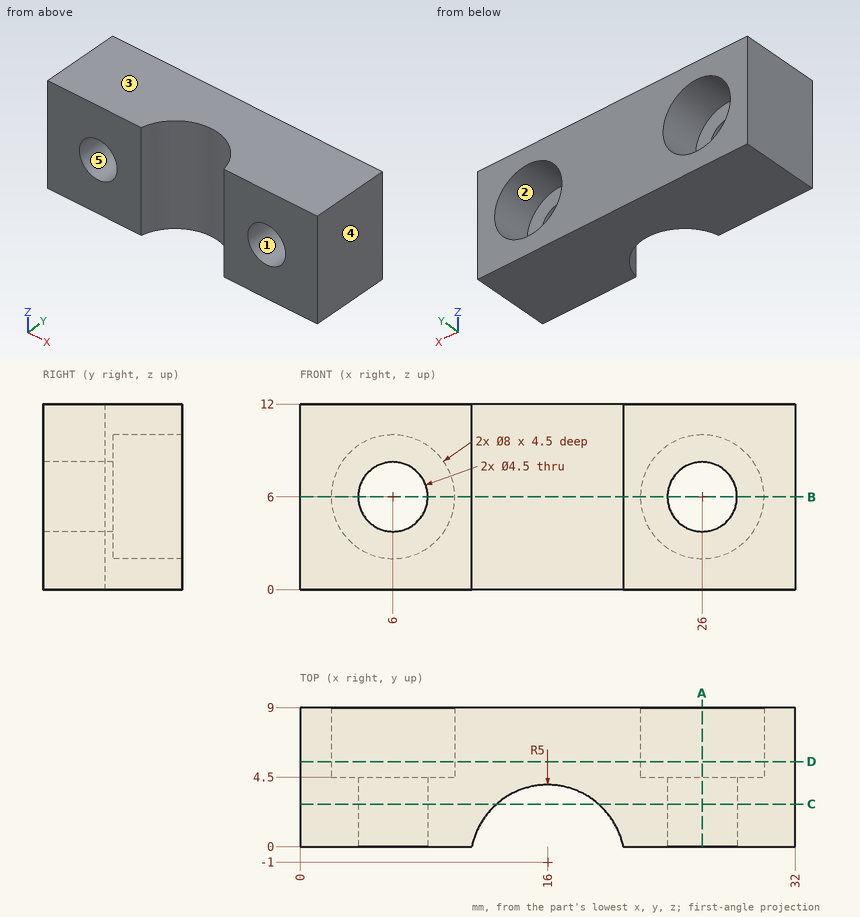
Geometry check sheet. Reference: drawing and pictorial views, mm from the part's lowest x, y, z. A direction names the side the tool comes from. Coordinates: 2 decimals unless noted, no trailing zeros. Write each loop counter-clockwise with the first axis right and the second up, starting at its lowest first coordinate (ties: lowest second). Pieces come first, ordered by that corner, then holes. Notation, with made-up numbers: (45.25, -27.5) - (74.25, -27.5) arc R19 cw to (74.25, -23.5) - close; hole circle Ø11 at (34.5, 32). An arc over 180 degrees is marked (long way). One line per question, with ' | ' between items. Start each with the question number.
1. Gauge pin test, flat end, axial feed: P1, Ø2.5, axis at x = 28, z = 5, coming from the +Y side. Record the tip position at first contact, or that the pin passes through.
2. Draft check along Z on the marked faces 3, 4 and 5. Enter one of: released by +Z, released by -Z, zero draft, split by the parting line, or undercut.
3. Access from +Z, -Z, +X, -X, +Y, -Y to the whole of each face (thin tool, end or side, straight path). Record for the marked faces 1 and 2.
4. Section check A-A (x = 26). Enter the section's corners in (y, z), plus the area to 4 significant figures.
5. Section check C-C (y = 2.75). Enter the section's corners in (x, z), plus the area to 3 significant figures.
6. Section check D-D (y = 5.5). Enter the section's corners in (x, z), plus the area to 3 significant figures.
7. Section check B-B (z = 6). Enter the section's corners in (x, y).
8. Material ranges on line 1 along X through (y, z) = (5.9, 6); line 2 along Z through (x, y) = (6, 2.75); line 3 along Z through (x, y) = (6, 6.75), recorded low to high.
Computed values:
1) P1: y = 4.5
2) face 3: released by +Z | face 4: zero draft | face 5: undercut
3) face 1: +Y, -Y | face 2: +Y
4) outline: (0, 0) - (9, 0) - (9, 2) - (4.5, 2) - (4.5, 3.75) - (0, 3.75) - close; (0, 8.25) - (4.5, 8.25) - (4.5, 10) - (9, 10) - (9, 12) - (0, 12) - close | area: 51.75 mm²
5) outline: (0, 0) - (12.69, 0) - (12.69, 12) - (0, 12) - close; (19.31, 0) - (32, 0) - (32, 12) - (19.31, 12) - close; hole circle Ø4.5 at (6, 6); hole circle Ø4.5 at (26, 6) | area: 273 mm²
6) outline: (0, 0) - (32, 0) - (32, 12) - (0, 12) - close; hole circle Ø8 at (6, 6); hole circle Ø8 at (26, 6) | area: 283 mm²
7) outline: (0, 0) - (3.75, 0) - (3.75, 4.5) - (2, 4.5) - (2, 9) - (0, 9) - close; (8.25, 0) - (11.1, 0) arc R5 cw to (20.9, 0) - (23.75, 0) - (23.75, 4.5) - (22, 4.5) - (22, 9) - (10, 9) - (10, 4.5) - (8.25, 4.5) - close; (28.25, 0) - (32, 0) - (32, 9) - (30, 9) - (30, 4.5) - (28.25, 4.5) - close
8) line 1: 0 to 2, 10 to 22, 30 to 32 | line 2: 0 to 3.75, 8.25 to 12 | line 3: 0 to 2, 10 to 12
